Check sheet for the drawn part. Datum: minimum x, y, z corner. Units: mm. A direction names the side the tool comes from. Round coordinates to 2 decimals unless told otherwise and drop trailing zeros. Write each loop counter-clockwise with the first axis right and the second up, starting at its lowest first coordinate (ties: lowest second). Pieces come first, ordered by that corner, then holes.
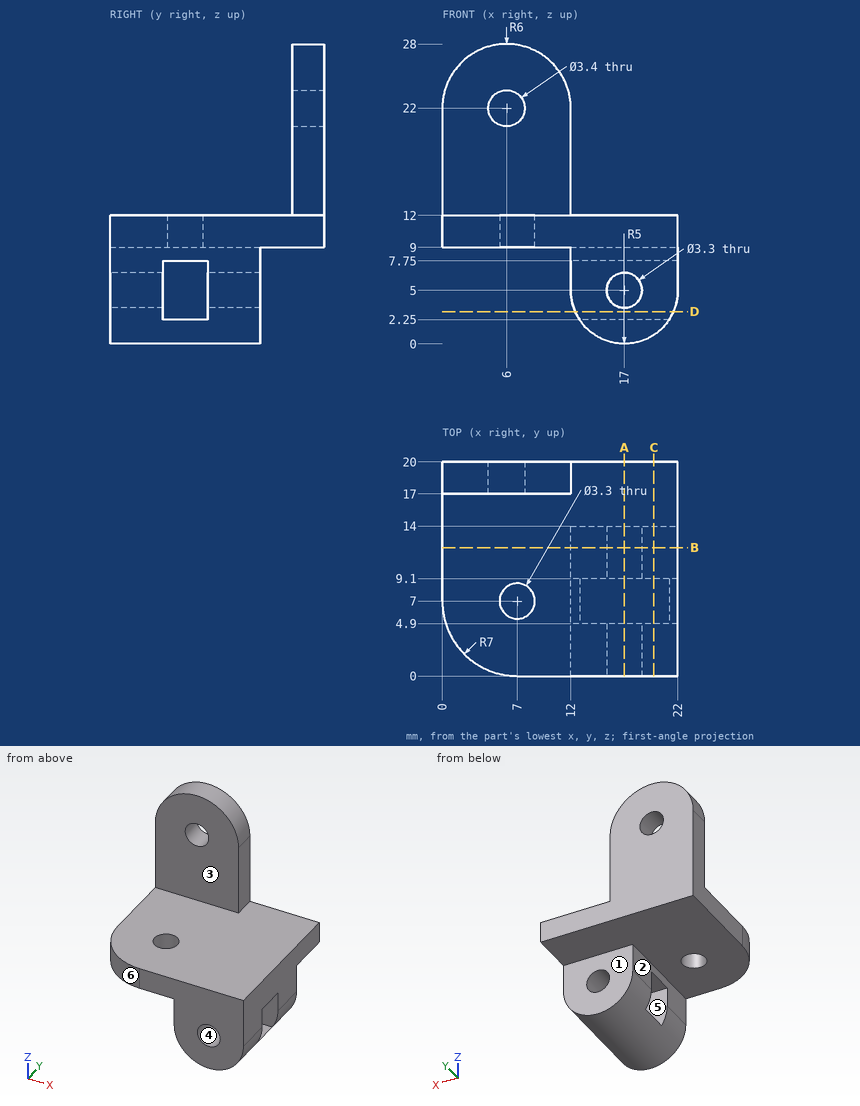
Q1. Material ranges on line 1 along Y through (x, z) = (7, 9.8); line 2 along Z through (x, y) = (17, 12.35); line 3 along Z through (x, y) = (6, 19.05), recorded low to high.
Recorded:
line 1: y = 0 to 5.35, 8.65 to 20
line 2: z = 0 to 3.35, 6.65 to 12
line 3: z = 9 to 20.3, 23.7 to 28
Q2. Tool access check on the marked faces 1, 2 and 3. Record the directions out of +Z, -Z, +X, -X, +Y, -Y that give a thin tool (end or side, any length) a straight path to the whole face; none if there is none.
Recorded:
face 1: -Z, +X, -X, +Y
face 2: -Z, -X, +Y, -Y
face 3: +Z, +X, -X, -Y
Q3. Release check for a two-part mould opening along X. For the marked faces 4, 5 and 6 record: released by +X, released by -X, zero draft, split by the parting line, or undercut.
Recorded:
face 4: undercut
face 5: zero draft
face 6: released by -X
Q4. Depth check by flat-ended pin: P1, Ø1.7, axis at x = 14.5, z = 4.5, coming from the +Y side; P2, Ø2, axis at x = 7, y = 7, coming from the -Z side; P3, Ø1.3, axis at x = 15, y = 6.5, coming from the -Z side; P4, Ø6, axis at x = 16, y = 10.5, coming from the +Z side. Enter the tip coordinate at first touch or a pass-through.
Recorded:
P1: stops at y = 14
P2: passes through
P3: stops at z = 0.19
P4: stops at z = 12
Q5. Sectioned sample at B-B (y = 12). Enter the section's corners in (x, z), plus the area to 3 significant figures.
Recorded:
outline: (0, 9) - (12, 9) - (12, 5) arc R5 ccw to (22, 5) - (22, 12) - (0, 12) - close; hole circle Ø3.3 at (17, 5)
area: 137 mm2
Q6. Sectioned sample at A-A (x = 17). Enter the section's corners in (y, z).
Recorded:
outline: (0, 0) - (14, 0) - (14, 3.35) - (9.1, 3.35) - (9.1, 2.25) - (4.9, 2.25) - (4.9, 3.35) - (0, 3.35) - close; (0, 6.65) - (4.9, 6.65) - (4.9, 7.75) - (9.1, 7.75) - (9.1, 6.65) - (14, 6.65) - (14, 9) - (20, 9) - (20, 12) - (0, 12) - close
Q7. Sectioned sample at D-D (z = 3). Enter the section's corners in (x, y).
Recorded:
outline: (12.42, 0) - (21.58, 0) - (21.58, 4.9) - (12.42, 4.9) - close; (12.42, 9.1) - (21.58, 9.1) - (21.58, 14) - (12.42, 14) - close
Q8. Sectioned sample at C-C (x = 19.75). Enter the section's corners in (y, z).
Recorded:
outline: (0, 0.82) - (14, 0.82) - (14, 9) - (20, 9) - (20, 12) - (0, 12) - close; hole (4.9, 2.25) - (9.1, 2.25) - (9.1, 7.75) - (4.9, 7.75) - close
